```python
from build123d import *

# Parameters (mm, degrees)
F1_DEPTH = 6.35


with BuildPart() as f1:
    # F0 (on Right) → F1 (new body)
    with BuildSketch(Plane.YZ):
        with BuildLine():
            ThreePointArc((-28.955078, 0.731324), (-35.154588, -2.159556), (-38.045467, -8.359066))
            Line((-38.045467, -8.359066), (-50, -145))
            Line((-50, -145), (50, -145))
            Line((50, -145), (41.091779, -43.178569))
            ThreePointArc((41.091779, -43.178569), (43.393282, -35.879135), (50.182169, -32.345065))
            Line((50.182169, -32.345065), (261.544266, -13.853277))
            Line((261.544266, -13.853277), (329.379022, -13.853277))
            add(Edge.make_bspline(
                [(341.544266, 4.146723), (341.544266, -3.148999), (341.544266, -12.045636), (329.379022, -13.853277)],
                knots=[0, 0, 0, 0, 21.725403, 21.725403, 21.725403, 21.725403], degree=3))
            Line((341.544266, 4.146723), (341.544266, 26.146723))
            Line((341.544266, 26.146723), (261.544266, 26.146723))
            Line((261.544266, 26.146723), (-28.955078, 0.731324))
        make_face()
        with BuildLine():
            ThreePointArc((341.544266, 4.146723), (352.544266, 15.146723), (341.544266, 26.146723))
            Line((341.544266, 26.146723), (341.544266, 4.146723))
        make_face()
    extrude(amount=F1_DEPTH)


solid = f1.part
```
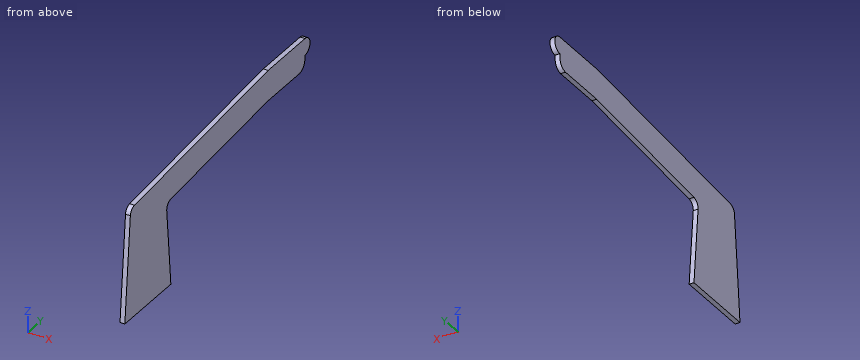
Source: CAD feature listing. Evaluate the final solid. Frame: model axes, mm. Round coordinates to 2 decimals unless told otherwise and drop trailing zeros. Loops run counter-clockwise (first coordinate to the right, second up) from the corner with the lowest first, then second, coordinate; pieces in that order, holes last.
1. Section query B-B on z = -100.5. Output: boundary loops of the cut face in (x, y).
2. Contact query for a flat-ended pin moving along its axis: pin 1 (5 mm diameter, centred on y = 27, z = -27.5, fed in from -X). Output: stop coordinate, or through.
3. Section query A-A on y = 323. Output: boundary loops of the cut face in (x, z).
4. Ray query, L1, parallel to Z at x = 5.5, y = -16; L2, parallel to Z at x = 1.5, y = 86.5; L3, parallel to Y at x = 1.5, z = -81. Return the intervals inside material, ascending.
Answers below:
1. outline: (0, -46.11) - (6.35, -46.11) - (6.35, 46.11) - (0, 46.11) - close
2. pin 1: stops at x = 0
3. outline: (0, -13.85) - (6.35, -13.85) - (6.35, 26.15) - (0, 26.15) - close
4. L1: z = -145 to 1.86
4. L2: z = -29.17 to 10.83
4. L3: y = -44.4 to 44.4
